```python
from build123d import *

# Parameters (mm, degrees)
F1_DEPTH       = 165.1
F3_D           = 8.7376
F3_CSINK_D     = 16.6624
F3_CSINK_ANGLE = 82
F4_W           = 6.35
F4_H           = 10.16
F5_DEPTH       = 2.54
F7_DEPTH       = 165.101


with BuildPart() as f1:
    # F0 (on Front) → F1 (new body)
    with BuildSketch(Plane.XZ):
        Polygon((0, 25.4), (0, 0), (6.35, 0), (6.35, 18.034), (3.2131, 18.034), (3.81, 25.4), align=None)
    extrude(amount=F1_DEPTH)

    # F3 (through all)
    with Locations(Plane(origin=(0, 0, 0), x_dir=(0, -1, 0), z_dir=(-1, 0, 0))):
        with Locations((19.05, 11.43), (146.05, 11.43)):
            CounterSinkHole(F3_D / 2, F3_CSINK_D / 2, counter_sink_angle=F3_CSINK_ANGLE)

    # F4 (on face) → F5 (join)
    with BuildSketch(Plane(origin=(0, 0, 0), x_dir=(1, 0, 0), z_dir=(0, 0, -1))):
        with Locations((3.175, 160.02)):
            Rectangle(F4_W, F4_H)
        with Locations((3.175, 5.08)):
            Rectangle(F4_W, F4_H)
    extrude(amount=F5_DEPTH)

    # F6 (on face) → F7 (cut, through all)
    with BuildSketch(Plane(origin=(0, 0, 0), x_dir=(-1, 0, 0), z_dir=(0, 1, 0))):
        Polygon((0, -1.4203236725), (-6.35, -2.54), (0, -2.54), align=None)
    extrude(amount=-F7_DEPTH, mode=Mode.SUBTRACT)


solid = f1.part
```
Check sheet for the modelled part. Datum: model origin and axes. Units: mm. A direction names the side the tool comes from. Coordinates: 2 decimals unless noted, no trailing zeros. Write each loop counter-clockwise with the first axis right and the second up, starting at its lowest first coordinate (ties: lowest second). Pieces come first, ordered by that corner, then holes. Notation, with made-up numbers: M -27.5,87.25 L 3.5,87.25 A17 cw 3.5,96.25 Z; hole C 67.5,4 d8. An arc over 180 degrees is marked long. Use one line per item in the form item = value.
Item 1: Sectioned sample at B-B, the plane x = 2.25. Record the cut outline in (y, z).
Answer below:
outline = M -165.1,-1.82 L -154.94,-1.82 L -154.94,0 L -10.16,0 L -10.16,-1.82 L 0,-1.82 L 0,25.4 L -165.1,25.4 Z; hole C -146.05,11.43 d12.75; hole C -19.05,11.43 d12.75
Item 2: Set-up check for faces 1 (the face through (3, -10.16, -1)), 2 (the face through (5.467, -150.415, 11.622)), 3 (the face through (5, -81, 18.034)): record each of +Z, -Z, +X, -X, +Y, -Y from which the full face is reachable in a straight line by a thin tool's end or side.
Answer below:
face_1 = -Z, +X, -X
face_2 = +X, -X
face_3 = +X, +Y, -Y
Item 3: Material ranges on L1, parallel to Y at x = 5.95, z = 11.43; L2, parallel to Y at x = 1.5, z = 10; L3, parallel to Z at x = 6.05, y = -19.05, recorded low to high. Write a range as from..to.
Answer below:
L1 = -165.1..-150.42, -141.68..-23.42, -14.68..0
L2 = -165.1..-152.93, -139.17..-25.93, -12.17..0
L3 = 0..7.06, 15.8..18.03
Item 4: Sectioned sample at A-A, the plane y = -146.05. Record the cut outline in (x, z), and give its area (3 significant figures).
Answer below:
outline = M 0,0 L 6.35,0 L 6.35,7.06 L 4.56,7.06 L 0,3.1 Z; M 0,19.76 L 4.56,15.8 L 6.35,15.8 L 6.35,18.03 L 3.21,18.03 L 3.81,25.4 L 0,25.4 Z
area = 66.8 mm^2
Item 5: Release check for a two-part mould opening along Z. For faces 4 (the face through (3, -82, 0)), 5 (the face through (3, -154.94, -1)), 6 (the face through (4.337, -149.67, 8.655)) record: pulls with the +Z half, pulls with the -Z half, needs draft (parallel to the pull), parting line crosses it, or undercut.
Answer below:
face_4 = pulls with the -Z half
face_5 = needs draft
face_6 = undercut
Item 6: Sectioned sample at C-C, the plane y = -71. Record the cut outline in (x, z), and give its area (3 significant figures).
Answer below:
outline = M 0,0 L 6.35,0 L 6.35,18.03 L 3.21,18.03 L 3.81,25.4 L 0,25.4 Z
area = 140 mm^2
Item 7: Gauge pin test, flat ends, axial feed: pin 1 Ø1.5 at (x, y) = (3.5, -101.5) entering from -Z; pin 2 Ø2 at (x, y) = (5.5, -140.5) entering from +Z. Record the tip position at first contact, or that the pin passes through.
Answer below:
pin_1 = 0
pin_2 = 18.03
